```python
from build123d import *

# Parameters (mm, degrees)
F0_R     = 40
F1_DEPTH = 2
F2_DEPTH = 1
F3_R     = 1
F4_DEPTH = 25


with BuildPart() as f1:
    # F0 (on Top) → F1 (new body)
    with BuildSketch(Plane.XY):
        Circle(F0_R)
        with BuildLine():
            ThreePointArc((-36.4644660941, -3.5355339059), (-16.4644660941, -23.5355339059), (3.5355339059, -3.5355339059))
            Line((3.5355339059, -3.5355339059), (5.7855339059, -3.5355339059))
            ThreePointArc((5.7855339059, -3.5355339059), (-16.4644660941, -25.7855339059), (-38.7144660941, -3.5355339059))
            Line((-38.7144660941, -3.5355339059), (-36.4644660941, -3.5355339059))
        make_face(mode=Mode.SUBTRACT)
        with BuildLine():
            ThreePointArc((3.5355339059, -36.4644660941), (23.5355339059, -16.4644660941), (3.5355339059, 3.5355339059))
            Line((3.5355339059, 3.5355339059), (3.5355339059, 5.7855339059))
            ThreePointArc((3.5355339059, 5.7855339059), (25.7855339059, -16.4644660941), (3.5355339059, -38.7144660941))
            Line((3.5355339059, -38.7144660941), (3.5355339059, -36.4644660941))
        make_face(mode=Mode.SUBTRACT)
        with BuildLine():
            ThreePointArc((-3.5355339059, 36.4644660941), (-23.5355339059, 16.4644660941), (-3.5355339059, -3.5355339059))
            Line((-3.5355339059, -3.5355339059), (-3.5355339059, -5.7855339059))
            ThreePointArc((-3.5355339059, -5.7855339059), (-25.7855339059, 16.4644660941), (-3.5355339059, 38.7144660941))
            Line((-3.5355339059, 38.7144660941), (-3.5355339059, 36.4644660941))
        make_face(mode=Mode.SUBTRACT)
        with BuildLine():
            ThreePointArc((3.5355339059, 3.5355339059), (4.6193976626, 1.9134171618), (5, 0))
            ThreePointArc((5, 0), (4.6193976626, -1.9134171618), (3.5355339059, -3.5355339059))
            ThreePointArc((3.5355339059, -3.5355339059), (0, -5), (-3.5355339059, -3.5355339059))
            ThreePointArc((-3.5355339059, -3.5355339059), (-5, 0), (-3.5355339059, 3.5355339059))
            ThreePointArc((-3.5355339059, 3.5355339059), (0, 5), (3.5355339059, 3.5355339059))
        make_face(mode=Mode.SUBTRACT)
        with BuildLine():
            ThreePointArc((36.4644660941, 3.5355339059), (16.4644660941, 23.5355339059), (-3.5355339059, 3.5355339059))
            Line((-3.5355339059, 3.5355339059), (-5.7855339059, 3.5355339059))
            ThreePointArc((-5.7855339059, 3.5355339059), (16.4644660941, 25.7855339059), (38.7144660941, 3.5355339059))
            Line((38.7144660941, 3.5355339059), (36.4644660941, 3.5355339059))
        make_face(mode=Mode.SUBTRACT)
        with BuildLine():
            Line((-3.5355339059, -5.7855339059), (-3.5355339059, -3.5355339059))
            ThreePointArc((-3.5355339059, -3.5355339059), (-23.5355339059, 16.4644660941), (-3.5355339059, 36.4644660941))
            Line((-3.5355339059, 36.4644660941), (-3.5355339059, 38.7144660941))
            ThreePointArc((-3.5355339059, 38.7144660941), (-25.7855339059, 16.4644660941), (-3.5355339059, -5.7855339059))
        make_face()
        with BuildLine():
            Line((5.7855339059, -3.5355339059), (3.5355339059, -3.5355339059))
            ThreePointArc((3.5355339059, -3.5355339059), (-16.4644660941, -23.5355339059), (-36.4644660941, -3.5355339059))
            Line((-36.4644660941, -3.5355339059), (-38.7144660941, -3.5355339059))
            ThreePointArc((-38.7144660941, -3.5355339059), (-16.4644660941, -25.7855339059), (5.7855339059, -3.5355339059))
        make_face()
        with BuildLine():
            Line((3.5355339059, 5.7855339059), (3.5355339059, 3.5355339059))
            ThreePointArc((3.5355339059, 3.5355339059), (23.5355339059, -16.4644660941), (3.5355339059, -36.4644660941))
            Line((3.5355339059, -36.4644660941), (3.5355339059, -38.7144660941))
            ThreePointArc((3.5355339059, -38.7144660941), (25.7855339059, -16.4644660941), (3.5355339059, 5.7855339059))
        make_face()
        with BuildLine():
            Line((-5.7855339059, 3.5355339059), (-3.5355339059, 3.5355339059))
            ThreePointArc((-3.5355339059, 3.5355339059), (16.4644660941, 23.5355339059), (36.4644660941, 3.5355339059))
            Line((36.4644660941, 3.5355339059), (38.7144660941, 3.5355339059))
            ThreePointArc((38.7144660941, 3.5355339059), (16.4644660941, 25.7855339059), (-5.7855339059, 3.5355339059))
        make_face()
        Polygon((0, 0), (3.5355339059, 3.5355339059), (-3.5355339059, 3.5355339059), align=None)
        with BuildLine():
            Line((-3.5355339059, 3.5355339059), (3.5355339059, 3.5355339059))
            ThreePointArc((3.5355339059, 3.5355339059), (0, 5), (-3.5355339059, 3.5355339059))
        make_face()
        Polygon((0, 0), (-3.5355339059, 3.5355339059), (-3.5355339059, -3.5355339059), align=None)
        Polygon((-3.5355339059, -3.5355339059), (3.5355339059, -3.5355339059), (0, 0), align=None)
        Polygon((3.5355339059, -3.5355339059), (3.5355339059, 3.5355339059), (0, 0), align=None)
        with BuildLine():
            ThreePointArc((3.5355339059, -3.5355339059), (4.6193976626, -1.9134171618), (5, 0))
            ThreePointArc((5, 0), (4.6193976626, 1.9134171618), (3.5355339059, 3.5355339059))
            Line((3.5355339059, 3.5355339059), (3.5355339059, -3.5355339059))
        make_face()
        with BuildLine():
            ThreePointArc((-3.5355339059, -3.5355339059), (0, -5), (3.5355339059, -3.5355339059))
            Line((3.5355339059, -3.5355339059), (-3.5355339059, -3.5355339059))
        make_face()
        with BuildLine():
            Line((-3.5355339059, -3.5355339059), (-3.5355339059, 3.5355339059))
            ThreePointArc((-3.5355339059, 3.5355339059), (-5, 0), (-3.5355339059, -3.5355339059))
        make_face()
    extrude(amount=F1_DEPTH)

    # F0 (on Top) → F2 (cut)
    with BuildSketch(Plane.XY):
        with BuildLine():
            Line((-5.7855339059, 3.5355339059), (-3.5355339059, 3.5355339059))
            ThreePointArc((-3.5355339059, 3.5355339059), (16.4644660941, 23.5355339059), (36.4644660941, 3.5355339059))
            Line((36.4644660941, 3.5355339059), (38.7144660941, 3.5355339059))
            ThreePointArc((38.7144660941, 3.5355339059), (16.4644660941, 25.7855339059), (-5.7855339059, 3.5355339059))
        make_face()
        with BuildLine():
            Line((3.5355339059, 5.7855339059), (3.5355339059, 3.5355339059))
            ThreePointArc((3.5355339059, 3.5355339059), (23.5355339059, -16.4644660941), (3.5355339059, -36.4644660941))
            Line((3.5355339059, -36.4644660941), (3.5355339059, -38.7144660941))
            ThreePointArc((3.5355339059, -38.7144660941), (25.7855339059, -16.4644660941), (3.5355339059, 5.7855339059))
        make_face()
        with BuildLine():
            Line((5.7855339059, -3.5355339059), (3.5355339059, -3.5355339059))
            ThreePointArc((3.5355339059, -3.5355339059), (-16.4644660941, -23.5355339059), (-36.4644660941, -3.5355339059))
            Line((-36.4644660941, -3.5355339059), (-38.7144660941, -3.5355339059))
            ThreePointArc((-38.7144660941, -3.5355339059), (-16.4644660941, -25.7855339059), (5.7855339059, -3.5355339059))
        make_face()
        with BuildLine():
            Line((-3.5355339059, -5.7855339059), (-3.5355339059, -3.5355339059))
            ThreePointArc((-3.5355339059, -3.5355339059), (-23.5355339059, 16.4644660941), (-3.5355339059, 36.4644660941))
            Line((-3.5355339059, 36.4644660941), (-3.5355339059, 38.7144660941))
            ThreePointArc((-3.5355339059, 38.7144660941), (-25.7855339059, 16.4644660941), (-3.5355339059, -5.7855339059))
        make_face()
    extrude(amount=F2_DEPTH, mode=Mode.SUBTRACT)

    # F3
    f3_edges = [f1.edges().sort_by_distance(p)[0] for p in [
        (-5.785534, 3.535534, 0.5),
        (-3.535534, 3.535534, 0.5),
        (-3.535534, -5.785534, 0.5),
        (-3.535534, -3.535534, 0.5),
        (5.785534, -3.535534, 0.5),
        (3.535534, -3.535534, 0.5),
        (3.535534, 5.785534, 0.5),
        (3.535534, 3.535534, 0.5),
        (3.535534, -38.714466, 0.5),
        (3.535534, -36.464466, 0.5),
        (-38.714466, -3.535534, 0.5),
        (-36.464466, -3.535534, 0.5),
        (-3.535534, 38.714466, 0.5),
        (-3.535534, 36.464466, 0.5),
        (38.714466, 3.535534, 0.5),
        (36.464466, 3.535534, 0.5),
    ]]
    fillet(f3_edges, radius=F3_R)

    # F0 (on Top) → F4 (cut)
    with BuildSketch(Plane.XY):
        Polygon((3.5355339059, -3.5355339059), (3.5355339059, 3.5355339059), (0, 0), align=None)
        with BuildLine():
            ThreePointArc((3.5355339059, -3.5355339059), (4.6193976626, -1.9134171618), (5, 0))
            ThreePointArc((5, 0), (4.6193976626, 1.9134171618), (3.5355339059, 3.5355339059))
            Line((3.5355339059, 3.5355339059), (3.5355339059, -3.5355339059))
        make_face()
        Polygon((-3.5355339059, -3.5355339059), (3.5355339059, -3.5355339059), (0, 0), align=None)
        with BuildLine():
            ThreePointArc((-3.5355339059, -3.5355339059), (0, -5), (3.5355339059, -3.5355339059))
            Line((3.5355339059, -3.5355339059), (-3.5355339059, -3.5355339059))
        make_face()
        Polygon((0, 0), (-3.5355339059, 3.5355339059), (-3.5355339059, -3.5355339059), align=None)
        Polygon((0, 0), (3.5355339059, 3.5355339059), (-3.5355339059, 3.5355339059), align=None)
        with BuildLine():
            Line((-3.5355339059, 3.5355339059), (3.5355339059, 3.5355339059))
            ThreePointArc((3.5355339059, 3.5355339059), (0, 5), (-3.5355339059, 3.5355339059))
        make_face()
        with BuildLine():
            Line((-3.5355339059, -3.5355339059), (-3.5355339059, 3.5355339059))
            ThreePointArc((-3.5355339059, 3.5355339059), (-5, 0), (-3.5355339059, -3.5355339059))
        make_face()
    extrude(amount=F4_DEPTH, mode=Mode.SUBTRACT)


solid = f1.part
```
The model under review builds one solid part; all positions refer to its coordinate system, in mm. A direction names the side the tool comes from. Round coordinates to 2 decimals unless told otherwise and drop trailing zeros. Loops run counter-clockwise (first coordinate to the right, second up) from the corner with the lowest first, then second, coordinate; pieces in that order, holes last. Notation, with made-up numbers: M -19.75,-12.5 L 23.25,-12.5 A24 ccw 23.25,15.5 Z; hole C 71.25,77.25 d8. An arc over 180 degrees is marked long. Write item = value, one per line.
Item 1: Take a section at A-A on z = 1.7. Write out the cut boundary in (x, y), then the cut area to 3 significant figures.
Return value:
outline = C 0,0 d80; hole C 0,0 d10
area = 4,950 mm2
Item 2: Take a section at D-D on x = 0. Write out the cut boundary in (y, z).
Return value:
outline = M -40,0 L -18.5,0 L -18.5,1 L -14.89,1 L -14.89,0 L -5,0 L -5,2 L -40,2 Z; M 5,0 L 14.89,0 L 14.89,1 L 18.5,1 L 18.5,0 L 40,0 L 40,2 L 5,2 Z
Item 3: Insertion check: P1, Ø8, axis at x = 29, y = 6, coming from the -Z side; P2, Ø1, axis at y = 22, z = 0, coming from the -X side. Each pin has a flat end and moves straight along its axis. Give the tip position at first contact, or say it passes through.
Return value:
P1 = 0
P2 = -33.73
Item 4: Take a section at B-B on y = 8.5. Write out the cut boundary in (x, z).
Return value:
outline = M -39.09,0 L -24.31,0 L -24.31,1 L -21.88,1 L -21.88,0 L -5.22,0 L -5.22,1 L -2.91,1 L -2.91,0 L 35.84,0 L 35.84,1 L 38.15,1 L 38.15,0 L 39.09,0 L 39.09,2 L -39.09,2 Z
Item 5: The part is to be moulded in two halves that separate along X. For faces 1 (the cylindrical face through (-8.67, -39.05, 0.99)), 2 (the flat face through (16, 24, 1)), 3 (the flat face through (8, 1, 2)), 4 (the cylindrical face through (25.78, -16.94, 0.49)), say which applies: released by +X, released by -X, zero draft, split by the parting line, or undercut.
Return value:
face_1 = split by the parting line
face_2 = undercut
face_3 = zero draft
face_4 = undercut
Item 6: Take a section at C-C on x = -29.5. Write out the cut boundary in (y, z), then the cut area to 3 significant figures.
Return value:
outline = M -27.01,0 L -21.57,0 L -21.57,1 L -18.7,1 L -18.7,0 L 27.01,0 L 27.01,2 L -27.01,2 Z
area = 105 mm2
Item 7: For line 1 (X direction, y = 10, z = 0.8); line 2 (Y direction, x = 0, z = 1.6); line 3 (X direction, y = 11, z = 0.9) (3 decimals), list the stretches that pass through material, from the lowest coordinate up. Write a range as [from, to].
Return value:
line_1 = [-38.73, -24.83], [-22.46, -4.83], [-2.46, 35.39], [37.75, 38.73]
line_2 = [-40, -5], [5, 40]
line_3 = [-38.458, -25.104], [-22.775, -4.496], [-2.09, 35.019], [37.425, 38.458]
Item 8: Machinability: for faces 5 (the flat face through (8, 1, 0)), 6 (the cylindrical face through (-25.78, 16.94, 0.49)), which of the approach directions +Z, -Z, +X, -X, +Y, -Y give a long, thin tool a straight path to every point of the face, cutting with its end or side? Answer none if there is none.
Return value:
face_5 = -Z, +X, -X, +Y, -Y
face_6 = -Z
